The listing builds one solid part. Answer for the finished solid, in the listing's coordinates (mm). Face numbers are marked on the shaded views. A direction names the side the tool comes from. Give positions to 0.01 mm unless a question says otherwise; leave off trailing zeros. Order: outer loops, then holes, each group sorted by start corner. A loop starts at its lowest first (then second) coordinate and runs counter-clockwise, first axis right, second up. Notation, with made-up numbers: (83.25, 11.5) - (117.25, 11.5) arc R35 cw to (117.25, 48.5) - close; hole circle Ø5 at (4.25, 17). An arc over 180 degrees is marked (long way). Answer in a Markdown table with one row per item.
from build123d import *

# Parameters (mm, degrees)
SKETCH_1_R          = 8
EXTRUDE_1_DEPTH     = 1
SKETCH_2_R          = 6
EXTRUDE_2_DEPTH     = 7.5
SKETCH_3_R          = 8
EXTRUDE_3_DEPTH     = 0.5
CUT_EXTRUDE_1_REACH = 16.457
SKETCH_4_R          = 2.5


with BuildPart() as part:
    # 草图1 → 凸台-拉伸1 (new body)
    with BuildSketch(Plane(origin=(0, 0, 0), x_dir=(1, 0, 0), z_dir=(0, 1, 0))):
        with Locations(Location((0, 0, 0), (0, 0, 270))):
            Circle(SKETCH_1_R)
    extrude(amount=EXTRUDE_1_DEPTH)

    # 草图2 → 凸台-拉伸2 (add)
    with BuildSketch(Plane(origin=(0, 1, 0), x_dir=(1, 0, 0), z_dir=(0, 1, 0))):
        with Locations(Location((0, 0, 0), (0, 0, 270))):
            Circle(SKETCH_2_R)
    extrude(amount=EXTRUDE_2_DEPTH)

    # 草图3 → 凸台-拉伸3 (add)
    with BuildSketch(Plane(origin=(0, 8.5, 0), x_dir=(1, 0, 0), z_dir=(0, 1, 0))):
        with Locations(Location((0, 0, 0), (0, 0, 270))):
            Circle(SKETCH_3_R)
    extrude(amount=EXTRUDE_3_DEPTH)

    # 草图4 → 切除-拉伸1 (cut, up to next)
    with BuildSketch(Plane.XZ, mode=Mode.PRIVATE) as cut_extrude_1_sk1:
        with Locations(Location((0, 0, 0), (0, 0, 270))):
            Circle(SKETCH_4_R)
    cut_extrude_1_tool1 = extrude(cut_extrude_1_sk1.sketch, amount=-CUT_EXTRUDE_1_REACH, mode=Mode.PRIVATE) & part.part
    add(cut_extrude_1_tool1.solids().sort_by_distance((0, 0, 0))[0], mode=Mode.SUBTRACT)


solid = part.part
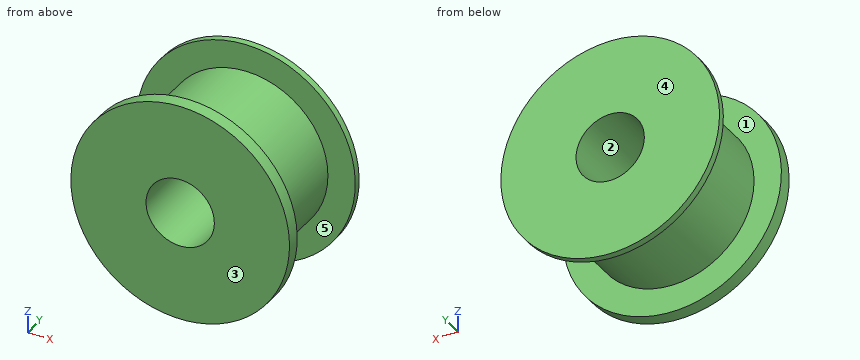
Item 1: Find section D-D on z = -4.5. Write down the section's boundary in (x, y).
Answer block:
| item | result |
|---|---|
| outline | (-6.61, 0) - (6.61, 0) - (6.61, 1) - (3.97, 1) - (3.97, 8.5) - (6.61, 8.5) - (6.61, 9) - (-6.61, 9) - (-6.61, 8.5) - (-3.97, 8.5) - (-3.97, 1) - (-6.61, 1) - close |
Item 2: Find section C-C on y = 6.5. Write down the section's boundary in (x, z), then the cut area to 3 significant figures.
Answer block:
| item | result |
|---|---|
| outline | circle Ø12 at (0, 0); hole circle Ø5 at (0, 0) |
| area | 93.5 mm² |
Item 3: Consider line 1 (Y direction, x = -5.5, z = -5.5); line 2 (X direction, y = 7, z = 0); line 3 (Z direction, x = 0.75, y = 2). Determine where each line is inside the solid, lowest interval first.
Answer block:
| item | result |
|---|---|
| line 1 | 0 to 1, 8.5 to 9 |
| line 2 | -6 to -2.5, 2.5 to 6 |
| line 3 | -5.95 to -2.38, 2.38 to 5.95 |
Item 4: Find section A-A on x = 0. Write down the section's boundary in (y, z).
Answer block:
| item | result |
|---|---|
| outline | (0, -8) - (1, -8) - (1, -6) - (8.5, -6) - (8.5, -8) - (9, -8) - (9, -2.5) - (0, -2.5) - close; (0, 2.5) - (9, 2.5) - (9, 8) - (8.5, 8) - (8.5, 6) - (1, 6) - (1, 8) - (0, 8) - close |
Item 5: Determine the mould class of the marked faces 1, 2 and 3 for opening direction Y: pulls with the +Y half, pulls with the -Y half, needs draft (parallel to the pull), parting line crosses it, or undercut.
Answer block:
| item | result |
|---|---|
| face 1 | undercut |
| face 2 | needs draft |
| face 3 | pulls with the -Y half |
Item 6: Which of the six approach directions +Z, -Z, +X, -X, +Y, -Y give full straight-line access (tool end or side, diameter ignored) to the marked faces 4 and 5?
Answer block:
| item | result |
|---|---|
| face 4 | +Z, -Z, +X, -X, +Y |
| face 5 | none |
Item 7: Find section B-B on z = 0. Write down the section's boundary in (x, y), then the cut area to 3 significant figures.
Answer block:
| item | result |
|---|---|
| outline | (-8, 0) - (-2.5, 0) - (-2.5, 9) - (-8, 9) - (-8, 8.5) - (-6, 8.5) - (-6, 1) - (-8, 1) - close; (2.5, 0) - (8, 0) - (8, 1) - (6, 1) - (6, 8.5) - (8, 8.5) - (8, 9) - (2.5, 9) - close |
| area | 69.0 mm² |
